from build123d import *

# Parameters (mm, degrees)
SKETCH_1_W          = 81
SKETCH_1_H          = 40
EXTRUDE_1_DEPTH     = 5
SKETCH_2_R          = 1.6
CUT_EXTRUDE_1_DEPTH = 6
FILLET_1_R          = 5
SKETCH_3_R          = 1.6
CUT_EXTRUDE_2_DEPTH = 6
CUT_EXTRUDE_5_DEPTH = 10
FILLET_2_R          = 5
FILLET_3_R          = 5
FILLET_4_R          = 1
FILLET_5_R          = 1


with BuildPart() as part:
    # 草图1 → 凸台-拉伸1 (new body)
    with BuildSketch(Plane(origin=(0, 0, 0), x_dir=(1, 0, 0), z_dir=(0, 1, 0))):
        Rectangle(SKETCH_1_W, SKETCH_1_H)
    extrude(amount=EXTRUDE_1_DEPTH)

    # 草图2 → 切除-拉伸1 (cut, through all)
    with BuildSketch(Plane.XZ):
        with Locations((36.75, 0)):
            Circle(SKETCH_2_R)
        with Locations((-1.75, 0)):
            Circle(SKETCH_2_R)
    extrude(amount=-CUT_EXTRUDE_1_DEPTH, mode=Mode.SUBTRACT)

    # 圆角1
    fillet_1_edges = [part.edges().sort_by_distance(p)[0] for p in [
        (40.5, 2.5, 20),
        (40.5, 2.5, -20),
    ]]
    fillet(fillet_1_edges, radius=FILLET_1_R)

    # 草图3 → 切除-拉伸2 (cut, through all)
    with BuildSketch(Plane.XZ):
        with Locations((-37.5, 5)):
            Circle(SKETCH_3_R)
        with Locations((-37.5, -15)):
            Circle(SKETCH_3_R)
    extrude(amount=-CUT_EXTRUDE_2_DEPTH, mode=Mode.SUBTRACT)

    # 草图4 → 切除-拉伸5 (cut)
    with BuildSketch(Plane.XZ):
        Polygon((32.5, 16), (-28.316233007, 16), (32.5, 1.029850337), align=None)
        with BuildLine():
            Line((-3.40399678, 4.718505553), (-32.5, 11.880598653))
            Line((-32.5, 11.880598653), (-32.5, 2.5))
            Line((-32.5, 2.5), (-6.080127019, 2.5))
            ThreePointArc((-6.080127019, 2.5), (-4.941061913, 3.849301738), (-3.40399678, 4.718505553))
        make_face()
        Polygon((32.5, -1.029850337), (-28.316233007, -16), (32.5, -16), align=None)
        with BuildLine():
            Line((15.764932029, 0), (1.905256588, 3.411612416))
            ThreePointArc((1.905256588, 3.411612416), (3.25, 0), (1.905256588, -3.411612416))
            Line((1.905256588, -3.411612416), (15.764932029, 0))
        make_face()
        with BuildLine():
            Line((-32.5, -2.5), (-32.5, -11.880598653))
            Line((-32.5, -11.880598653), (-3.40399678, -4.718505553))
            ThreePointArc((-3.40399678, -4.718505553), (-4.941061913, -3.849301738), (-6.080127019, -2.5))
            Line((-6.080127019, -2.5), (-32.5, -2.5))
        make_face()
    extrude(amount=-CUT_EXTRUDE_5_DEPTH, mode=Mode.SUBTRACT)

    # 圆角2
    fillet_2_edges = [part.edges().sort_by_distance(p)[0] for p in [
        (32.5, 2.5, 1.029850337),
        (32.5, 2.5, -1.029850337),
    ]]
    fillet(fillet_2_edges, radius=FILLET_2_R)

    # 圆角3
    fillet_3_edges = [part.edges().sort_by_distance(p)[0] for p in [
        (32.5, 2.5, 16),
        (32.5, 2.5, -16),
    ]]
    fillet(fillet_3_edges, radius=FILLET_3_R)

    # 圆角4
    fillet_4_edges = [part.edges().sort_by_distance(p)[0] for p in [
        (1.905256588, 2.5, -3.411612416),
        (1.905256588, 2.5, 3.411612416),
        (15.764932029, 2.5, 0),
    ]]
    fillet(fillet_4_edges, radius=FILLET_4_R)

    # 圆角5
    fillet_5_edges = [part.edges().sort_by_distance(p)[0] for p in [
        (-6.080127019, 2.5, -2.5),
        (-3.40399678, 2.5, -4.718505553),
        (-32.5, 2.5, -11.880598653),
        (-32.5, 2.5, -2.5),
        (-28.316233007, 2.5, 16),
        (-28.316233007, 2.5, -16),
        (-3.40399678, 2.5, 4.718505553),
        (-6.080127019, 2.5, 2.5),
        (-32.5, 2.5, 2.5),
        (-32.5, 2.5, 11.880598653),
    ]]
    fillet(fillet_5_edges, radius=FILLET_5_R)


solid = part.part
The model under review builds one solid part; all positions refer to its coordinate system, in mm. A direction names the side the tool comes from. Give positions to 0.01 mm unless a question says otherwise; leave off trailing zeros. Write each loop counter-clockwise with the first axis right and the second up, starting at its lowest first coordinate (ties: lowest second). Pieces come first, ordered by that corner, then holes.
1. Tool access review of faces 1 (the cylindrical face through (39, 2.54, -18.57)), 2 (the flat face through (3.324, 2.465, -8.212)): name each direction out of +Z, -Z, +X, -X, +Y, -Y from which nothing blocks a thin tool from reaching the whole face with its end or side.
2. Add section C-C, the plane x = 36.75. Write out the cut boundary in (y, z).
3. Add section A-A, the plane z = 0. Write out the cut boundary in (x, y).
4. Add section D-D, the plane z = -12.5. Write out the cut boundary in (x, y), plus the area to 3 significant figures.
5. Wall thickness on L1, parallel to Z at x = -37.5, y = 2.85; L2, parallel to Z at x = -7.5, y = 3.3; L3, parallel to Z at x = -16, y = 4.7: over which ranges is each line inside the solid? List them lowest first.
6. Add section B-B, the plane x = -37.5. Write out the cut boundary in (y, z).
7. Draft analysis for pull direction Z (two halves, no side actions). For faces 3 (the flat face through (-18.65, 2.46, -8.47)), 4 (the flat face through (-3, 2, -20)), 5 (the flat face through (-1, 0, 4)), state which applies: +Z half, -Z half, draft (parallel to the pull), parting line (faces both ways), or undercut.
Worked answers:
1. face 1: -Z, +X, +Y, -Y
1. face 2: +Y, -Y
2. outline: (0, -19.84) - (5, -19.84) - (5, -1.6) - (0, -1.6) - close; (0, 1.6) - (5, 1.6) - (5, 19.84) - (0, 19.84) - close
3. outline: (-40.5, 0) - (-3.35, 0) - (-3.35, 5) - (-40.5, 5) - close; (-0.15, 0) - (3.25, 0) - (3.25, 5) - (-0.15, 5) - close; (12.58, 0) - (35.15, 0) - (35.15, 5) - (12.58, 5) - close; (38.35, 0) - (40.5, 0) - (40.5, 5) - (38.35, 5) - close
4. outline: (-40.5, 0) - (-14.1, 0) - (-14.1, 5) - (-40.5, 5) - close; (32.27, 0) - (40.5, 0) - (40.5, 5) - (32.27, 5) - close
4. area: 173 mm2
5. L1: z = -20 to -16.6, -13.4 to 3.4, 6.6 to 20
5. L2: z = -20 to -16, -10.88 to -5.73, -2.5 to 2.5, 5.73 to 10.88, 16 to 20
5. L3: z = -20 to -16, -12.97 to -7.82, -2.5 to 2.5, 7.82 to 12.97, 16 to 20
6. outline: (0, -20) - (5, -20) - (5, -16.6) - (0, -16.6) - close; (0, -13.4) - (5, -13.4) - (5, 3.4) - (0, 3.4) - close; (0, 6.6) - (5, 6.6) - (5, 20) - (0, 20) - close
7. face 3: undercut
7. face 4: -Z half
7. face 5: draft
